```python
from build123d import *

# Parameters (mm, degrees)
SKETCH1_R           = 1.5
BOSS_EXTRUDE1_DEPTH = 1.83
FILLET1_R           = 1


with BuildPart() as part:
    # Sketch1 → Boss-Extrude1 (new, symmetric)
    # profile 1 of 3: a face of its own
    with BuildSketch(Plane.XY):
        with BuildLine():
            ThreePointArc((-12, 0), (-12.085474, 0.768774), (-12.337722, 1.5))
            ThreePointArc((-12.337722, 1.5), (-19, 0), (-12.337722, -1.5))
            ThreePointArc((-12.337722, -1.5), (-12.085474, -0.768774), (-12, 0))
        make_face()
        with Locations((-15.5, 0)):
            Circle(SKETCH1_R, mode=Mode.SUBTRACT)
    # profile 2 of 3: a face of its own
    with BuildSketch(Plane.XY):
        with BuildLine():
            Line((12.337722, 1.5), (-12.337722, 1.5))
            ThreePointArc((-12.337722, 1.5), (-12.085474, 0.768774), (-12, 0))
            ThreePointArc((-12, 0), (-12.085474, -0.768774), (-12.337722, -1.5))
            Line((-12.337722, -1.5), (12.337722, -1.5))
            ThreePointArc((12.337722, -1.5), (12, 0), (12.337722, 1.5))
        make_face()
    # profile 3 of 3: a face of its own
    with BuildSketch(Plane.XY):
        with BuildLine():
            ThreePointArc((19, 0), (16.268774, 3.414526), (12.337722, 1.5))
            ThreePointArc((12.337722, 1.5), (12, 0), (12.337722, -1.5))
            ThreePointArc((12.337722, -1.5), (16.268774, -3.414526), (19, 0))
        make_face()
        with Locations((15.5, 0)):
            Circle(SKETCH1_R, mode=Mode.SUBTRACT)
    extrude(amount=BOSS_EXTRUDE1_DEPTH, both=True)

    # Fillet1
    fillet1_edges = [part.edges().sort_by_distance(p)[0] for p in [
        (-12.337722, 1.5, 0),
        (12.337722, 1.5, 0.915),
        (12.337722, -1.5, 0.915),
        (-12.337722, -1.5, 0),
    ]]
    fillet(fillet1_edges, radius=FILLET1_R)


solid = part.part
```
Source: CAD feature listing. Evaluate the final solid. Frame: model axes, mm. A direction names the side the tool comes from. Coordinates: 2 decimals unless noted, no trailing zeros. Write each loop counter-clockwise with the first axis right and the second up, starting at its lowest first coordinate (ties: lowest second). Pieces come first, ordered by that corner, then holes. Notation, with made-up numbers: (73, -11.5) - (85, -11.5) arc R27 cw to (85, 14.5) - close; hole circle Ø5 at (65.25, 38). An arc over 180 degrees is marked (long way). Answer as a JSON object with one key per item and string values.
Q1. Draft query along X for faces 4 (the flat face through (0, 0, -1.83)), 5 (the cylindrical face through (12.236, 1.621, 0.026)). Return one class per face: released by +X, released by -X, zero draft, split by the parting line, or undercut.
Ans:
{"face 4": "zero draft", "face 5": "undercut"}
Q2. Section query D-D, the plane y = 2.75. Output: boundary loops of the cut face in (x, z).
Ans:
{"outline": "(-17.67, -1.83) - (-13.33, -1.83) - (-13.33, 1.83) - (-17.67, 1.83) - close; (13.33, -1.83) - (17.67, -1.83) - (17.67, 1.83) - (13.33, 1.83) - close"}
Q3. Set-up query: faces 1 (the flat face through (0, 1.5, 0)), 2 (the flat face through (0, 0, 1.83)), 3 (the cylindrical face through (-12.224, -1.615, -0.026)). Return all of +Z, -Z, +X, -X, +Y, -Y with unobstructed straight access to the full face (end or side cutting, diameter ignored); none if empty.
Ans:
{"face 1": "+Z, -Z, +Y", "face 2": "+Z, +X, -X, +Y, -Y", "face 3": "+Z, -Z, -Y"}
Q4. Section query B-B, the plane x = -15.5. Output: boundary loops of the cut face in (y, z).
Ans:
{"outline": "(-3.5, -1.83) - (-1.5, -1.83) - (-1.5, 1.83) - (-3.5, 1.83) - close; (1.5, -1.83) - (3.5, -1.83) - (3.5, 1.83) - (1.5, 1.83) - close"}
Q5. Section query A-A, the plane z = -0.3. Output: boundary loops of the cut face in (x, y), plus the area to 3 significant figures.
Ans:
{"outline": "(-12.59, -1.94) arc R1 cw to (-11.76, -1.5) - (11.76, -1.5) arc R1 cw to (12.59, -1.94) arc R3.5 ccw (long way) to (12.59, 1.94) arc R1 cw to (11.76, 1.5) - (-11.76, 1.5) arc R1 cw to (-12.59, 1.94) arc R3.5 ccw (long way) to start; hole circle Ø3 at (-15.5, 0); hole circle Ø3 at (15.5, 0)", "area": "136 mm2"}
Q6. Material intervals for line 1 (X direction, y = -1.25, z = 1.15); line 2 (Y direction, x = -15.5, z = 0.05); line 3 (Y direction, x = 7.5, z = 1.6), sorted ascending. Write a range as [from, to].
Ans:
{"line 1": "x = [-18.77, -16.33], [-14.67, 14.67], [16.33, 18.77]", "line 2": "y = [-3.5, -1.5], [1.5, 3.5]", "line 3": "y = [-1.5, 1.5]"}
Q7. Section query C-C, the plane y = 1. Output: boundary loops of the cut face in (x, z).
Ans:
{"outline": "(-18.85, -1.83) - (-16.62, -1.83) - (-16.62, 1.83) - (-18.85, 1.83) - close; (-14.38, -1.83) - (14.38, -1.83) - (14.38, 1.83) - (-14.38, 1.83) - close; (16.62, -1.83) - (18.85, -1.83) - (18.85, 1.83) - (16.62, 1.83) - close"}
Q8. First-contact query: pin 1 Ø1.1 at (x, z) = (3, 0.5) entering from -Y; pin 2 Ø1 at (x, z) = (12, 0.5) entering from -Y. Flat tips, straight axial feed; report the tip coordinate or a pass-through.
Ans:
{"pin 1": "stops at y = -1.5", "pin 2": "stops at y = -1.83"}
